from build123d import *


with BuildPart() as part:
    # Sweep1: sweep along a path in Sketch2
    with BuildLine(Plane.XY) as sweep1_path:
        Line((-43, 2.5), (-17.5, 2.5))
        Line((-17.5, 2.5), (-15, 0))
        Line((-15, 0), (15, 0))
        Line((15, 0), (17.5, 2.5))
        Line((17.5, 2.5), (43, 2.5))
    # Sketch1 → Sweep1 (sweep)
    with BuildSketch(Plane(origin=(0, 0, 0), x_dir=(0, 0, -1), z_dir=(1, 0, 0))):
        Polygon((10.5, 0), (-10.5, 0), (-10.5, 2.5), (-7.5, 2.5), (-7.5, 5), (-4.5, 5), (-4.5, 2.5), (-1.5, 2.5), (-1.5, 5), (1.5, 5), (1.5, 2.5), (4.5, 2.5), (4.5, 5), (7.5, 5), (7.5, 2.5), (10.5, 2.5), align=None)
    sweep(path=sweep1_path.line, transition=Transition.RIGHT)


solid = part.part
Read the model definition and answer for the solid it produces. Units are mm, in the model's axes. A direction names the side the tool comes from. Coordinates: 2 decimals unless noted, no trailing zeros. Write each loop counter-clockwise with the first axis right and the second up, starting at its lowest first coordinate (ties: lowest second). Pieces come first, ordered by that corner, then holes. Notation, with made-up numbers: (61, 55) - (82, 55) arc R21 ccw to (82, 66) - close; hole circle Ø4 at (-30, 39). An arc over 180 degrees is marked (long way). One line per question, with ' | ' between items.
Q1. Consider L1, parallel to Z at x = 18.5, y = 5.75; L2, parallel to Y at x = 32, z = -8; L3, parallel to X at y = 7, z = 5.5. Determine where each line is inside the solid, lowest interval first. Write a range as [from, to].
Result set:
L1: [-7.5, -4.5], [-1.5, 1.5], [4.5, 7.5] | L2: [2.5, 5] | L3: [-43, -14.93], [14.93, 43]
Q2. Find section D-D, the plane y = 1.25. Write down the section's boundary in (x, z).
Result set:
outline: (-16.25, -10.5) - (16.25, -10.5) - (16.25, 10.5) - (-16.25, 10.5) - close
Q3. Find section A-A, the plane x = 23.5. Write down the section's boundary in (y, z), plus the area to 3 significant figures.
Result set:
outline: (2.5, -10.5) - (5, -10.5) - (5, -7.5) - (7.5, -7.5) - (7.5, -4.5) - (5, -4.5) - (5, -1.5) - (7.5, -1.5) - (7.5, 1.5) - (5, 1.5) - (5, 4.5) - (7.5, 4.5) - (7.5, 7.5) - (5, 7.5) - (5, 10.5) - (2.5, 10.5) - close | area: 75.0 mm^2
Q4. Find section C-C, the plane y = 6. Write down the section's boundary in (x, z).
Result set:
outline: (-43, -7.5) - (-13.93, -7.5) - (-13.93, -4.5) - (-43, -4.5) - close; (-43, -1.5) - (-13.93, -1.5) - (-13.93, 1.5) - (-43, 1.5) - close; (-43, 4.5) - (-13.93, 4.5) - (-13.93, 7.5) - (-43, 7.5) - close; (13.93, -7.5) - (43, -7.5) - (43, -4.5) - (13.93, -4.5) - close; (13.93, -1.5) - (43, -1.5) - (43, 1.5) - (13.93, 1.5) - close; (13.93, 4.5) - (43, 4.5) - (43, 7.5) - (13.93, 7.5) - close
Q5. Determine the mould class of faces 6 (the flat face through (1, 2, -10.5)), 7 (the flat face through (-15.197, 3.732, 2.979)), 8 (the flat face through (0, 2.5, 9)), 9 (the flat face through (43, 4, 0)) for opening direction X: +X half, -X half, draft (parallel to the pull), parting line (faces both ways), or undercut.
Result set:
face 6: draft | face 7: undercut | face 8: undercut | face 9: +X half
Q6. Each of these flat-tipped pins is pushed along its axis until it touches: P1, Ø0.9, axis at x = 2.5, z = -6.5, coming from the +Y side; P2, Ø0.9, axis at x = 6.5, z = 3, coming from the +Y side; P3, Ø2.5, axis at x = -10, y = 4.5, coming from the -Z side. Where does it stop, or does it pass through?
Result set:
P1: y = 5 | P2: y = 2.5 | P3: z = -7.5
Q7. For faces 1 (the flat face through (-14.16, 6.23, -6.02)), 2 (the flat face through (30, 5, -9)), 3 (the flat face through (1, 4, 1.5)), 4 (the flat face through (-15.197, 3.732, 8.979)), 5 (the flat face through (15.232, 3.768, -9.021)), determine the directions among +Z, -Z, +X, -X, +Y, -Y from which every point of the face is accessible in a straight line to the end or side of a thin tool.
Result set:
face 1: +Z, -Z, +Y | face 2: -Z, +X, -X, +Y | face 3: +Y | face 4: +Z, +Y | face 5: -Z, +Y
Q8. Find section B-B, the plane z = -5.25. Write down the section's boundary in (x, y).
Result set:
outline: (-43, 2.5) - (-17.5, 2.5) - (-15, 0) - (15, 0) - (17.5, 2.5) - (43, 2.5) - (43, 7.5) - (15.43, 7.5) - (12.93, 5) - (-12.93, 5) - (-15.43, 7.5) - (-43, 7.5) - close
